Can you work these out from the model? Positions are in its coordinate system, mm. A direction names the side the tool comes from. Give positions to 0.01 mm unless a question says otherwise; leave off trailing zeros. Write each loop counter-clockwise with the first axis right and the second up, starting at its lowest first coordinate (ties: lowest second). Pieces come first, ordered by that corner, then holes. Notation, with made-up numbers: (58.25, 84) - (117.25, 84) arc R17 ccw to (117.25, 95) - close; hole circle Ø11 at (-33, -32). An arc over 180 degrees is marked (long way). Return JSON: item names as keys, results as strings. Group by question number.
from build123d import *

# Parameters (mm, degrees)
F1_DEPTH = 44.45


with BuildPart() as f1:
    # F0 (on Front) → F1 (new body, symmetric)
    with BuildSketch(Plane.XZ):
        Polygon((12.4714, 22.6569566138), (12.4714, 22.1290275277), (7.429338686, 25.0400629846), (7.886538686, 25.3040275277), (7.886538686, 25.8319566138), (7.429338686, 26.0959211569), (6.972138686, 25.8319566138), (6.984838669, 25.2820305117), (0.0126999831, 29.3073966589), (-6.946738686, 25.3186922245), (-6.438738686, 25.0253982878), (-6.438738686, 24.4388104143), (-6.946738686, 24.1455164775), (-7.454738686, 24.4388104143), (-7.454738686, 25.0253982878), (-12.446, 22.1436922245), (-11.938, 21.8503982878), (-11.938, 21.2638104143), (-12.446, 20.9705164775), (-12.954, 21.2638104143), (-12.954, 21.8503982878), (-17.945261314, 18.9686922245), (-17.437261314, 18.6753982878), (-17.437261314, 18.0888104143), (-17.945261314, 17.7955164775), (-18.453261314, 18.0888104143), (-18.453261314, 18.6753982878), (-25.3873000169, 14.6426998215), (-25.3873000169, 6.5919675272), (-25.8572, 6.8779290861), (-26.3144, 6.6139645431), (-26.3144, 6.0860354569), (-25.8572, 5.8220709139), (-25.4, 6.0860354569), (-25.4, 0.2639645431), (-25.8572, 0.5279290861), (-26.3144, 0.2639645431), (-26.3144, -0.2639645431), (-25.8572, -0.5279290861), (-25.4, -0.2639645431), (-25.4, -6.0860354569), (-25.8572, -5.8220709139), (-26.3144, -6.0860354569), (-26.3144, -6.6139645431), (-25.8572, -6.8779290861), (-25.4, -6.6139645431), (-25.4, -14.6646968374), (-18.453261314, -18.6753982878), (-18.453261314, -18.0888104143), (-17.945261314, -17.7955164775), (-17.437261314, -18.0888104143), (-17.437261314, -18.6753982878), (-17.945261314, -18.9686922245), (-12.954, -21.8503982878), (-12.954, -21.2638104143), (-12.446, -20.9705164775), (-11.938, -21.2638104143), (-11.938, -21.8503982878), (-12.446, -22.1436922245), (-7.454738686, -25.0253982878), (-7.454738686, -24.4388104143), (-6.946738686, -24.1455164775), (-6.438738686, -24.4388104143), (-6.438738686, -25.0253982878), (-6.946738686, -25.3186922245), (0, -29.3293936748), (6.972138686, -25.3040275277), (6.972138686, -25.8319566138), (7.429338686, -26.0959211569), (7.886538686, -25.8319566138), (7.886538686, -25.3040275277), (7.429338686, -25.0400629846), (12.4714, -22.1290275277), (12.4714, -22.6569566138), (12.9286, -22.9209211569), (13.3858, -22.6569566138), (13.3858, -22.1290275277), (12.9286, -21.8650629846), (17.970661314, -18.9540275277), (17.970661314, -19.4819566138), (18.427861314, -19.7459211569), (18.885061314, -19.4819566138), (18.885061314, -18.9540275277), (18.427861314, -18.6900629846), (25.4, -14.6646968374), (25.4, -6.6432939367), (24.892, -6.9365878735), (24.384, -6.6432939367), (24.384, -6.0567060633), (24.892, -5.7634121265), (25.4, -6.0567060633), (25.4, -0.2932939367), (24.892, -0.5865878735), (24.384, -0.2932939367), (24.384, 0.2932939367), (24.892, 0.5865878735), (25.4, 0.2932939367), (25.4, 6.0567060633), (24.892, 5.7634121265), (24.384, 6.0567060633), (24.384, 6.6432939367), (24.892, 6.9365878735), (25.4, 6.6432939367), (25.4, 14.6646968374), (18.427861314, 18.6900629846), (18.885061314, 18.9540275277), (18.885061314, 19.4819566138), (18.427861314, 19.7459211569), (17.970661314, 19.4819566138), (17.970661314, 18.9540275277), (12.9286, 21.8650629846), (13.3858, 22.1290275277), (13.3858, 22.6569566138), (12.9286, 22.9209211569), align=None)
        Polygon((-6.946738686, 23.3829522811), (-5.7783387198, 24.057528316), (-5.7783387198, 25.230704063), (0.0126999831, 28.574161817), (6.667338669, 24.7321043803), (18.110361314, 18.1401368532), (24.7396000339, 14.3127440938), (24.7396000339, 7.6111639085), (23.7236000339, 7.024576035), (23.7236000339, 5.675423965), (24.7396000339, 5.0888360915), (24.7396000339, 1.2611639085), (23.7236000339, 0.674576035), (23.7236000339, -0.674576035), (24.7396000339, -1.2611639085), (24.7396000339, -5.0888360915), (23.7236000339, -5.675423965), (23.7236000339, -7.024576035), (24.7396000339, -7.6111639085), (24.7396000339, -14.3127440938), (18.110361314, -18.1401368532), (6.667338669, -24.7321043803), (0, -28.5668294784), (-5.7783387198, -25.230704063), (-5.7783387198, -24.057528316), (-6.946738686, -23.3829522811), (-7.962738686, -23.9695401546), (-11.2776000339, -22.055704063), (-11.2776000339, -20.882528316), (-12.446, -20.2079522811), (-13.462, -20.7945401546), (-16.7768613479, -18.880704063), (-16.7768613479, -17.707528316), (-17.945261314, -17.0329522811), (-18.961261314, -17.6195401546), (-24.765, -14.2687500619), (-24.765, -6.6139645431), (-24.7523000169, 6.5919675272), (-24.7523000169, 14.2760824006), (-18.961261314, 17.6195401546), (-17.945261314, 17.0329522811), (-16.7768613479, 17.707528316), (-16.7768613479, 18.880704063), (-13.462, 20.7945401546), (-12.446, 20.2079522811), (-11.2776000339, 20.882528316), (-11.2776000339, 22.055704063), (-7.962738686, 23.9695401546), align=None, mode=Mode.SUBTRACT)
    extrude(amount=F1_DEPTH, both=True)


solid = f1.part
1) On a 3-axis mill with a long thin cutter (end or side, diameter ignored), from which of +Z, -Z, +X, -X, +Y, -Y can I reach the whole of each face in a straight line? I mean faces 1 (the face through (25.4, -1, -11)), 2 (the face through (24.74, -1, 11)). Say none if no direction works.
2) We'd pull the mould along X, two halves only. Please class faces 3 (the face through (-17.8, -44.45, 17.5)), 4 (the face through (-15.48, -0.62, -20.39)), 5 (the face through (24.74, -1, 3)): pulls with the +X half, pulls with the -X half, needs draft (parallel to the pull), parting line crosses it, or undercut.
3) Will these pins go through, and if not, where does the flat tip stop? pin 1 Ø1 at (x, y) = (-18, -24.5) entering from -Z; pin 2 Ø3.5 at (y, z) = (-9, -11) entering from -X; pin 3 Ø0.6 at (y, z) = (21, 18.5) entering from +X.
4) I need wall thicknesses on line 1 along X through (y, z) = (19.5, 8); line 2 along X through (y, z) = (22.5, 18); line 3 along X through (y, z) = (35, -22.5). Which ranges of each line are inside material? Lowest first, please.
5) Imagine slicing it at A-A, the plane z = -12.5. Write out the boundary of the cut face in (x, y) (3 decimals), and give its area (3 significant figures).
6) Imagine slicing it at B-B, the plane x = 2. Write out the boundary of the cut face in (y, z).
Resolved:
{
 "1": {"face 1": "+Z, -Z, +X, +Y, -Y", "face 2": "+Y, -Y"},
 "2": {"face 3": "needs draft", "face 4": "pulls with the -X half", "face 5": "undercut"},
 "3": {"pin 1": "z = -19.23", "pin 2": "x = -25.4", "pin 3": "x = 19.28"},
 "4": {"line 1": "-25.39 to -24.75, 24.74 to 25.4", "line 2": "-19.61 to -18.3, -17.59 to -16.78, 18.35 to 19.62", "line 3": "-11.83 to -10.51, 10.54 to 11.83, 12.47 to 13.39"},
 "5": {"outline": "(-25.4, -44.45) - (-24.765, -44.45) - (-24.765, 44.45) - (-25.4, 44.45) - close; (24.74, -44.45) - (25.4, -44.45) - (25.4, 44.45) - (24.74, 44.45) - close", "area": "115 mm^2"},
 "6": {"outline": "(-44.45, -28.17) - (44.45, -28.17) - (44.45, -27.42) - (-44.45, -27.42) - close; (-44.45, 27.43) - (44.45, 27.43) - (44.45, 28.16) - (-44.45, 28.16) - close"}
}
